Can you work these out from the model? Positions are in its coordinate system, mm. Give positions to 0.01 mm unless a question says otherwise; leave off trailing zeros. Write each loop counter-clockwise with the first axis right and the second up, starting at its lowest first coordinate (ties: lowest second). Pieces come first, ordered by that corner, then holes. Notation, with made-up numbers: (-6, 84) - (-2, 84) arc R28 cw to (-2, 121) - close; hole circle Ø9 at (59.25, 24). An arc over 180 degrees is marked (long way). Return JSON: item names as keys, results as strings. Group by question number.
from build123d import *

# Parameters (mm, degrees)
ESBO_O1_W                = 120
ESBO_O1_H                = 190
RESSALTO_EXTRUS_O1_DEPTH = 2
ESBO_O2_R                = 1
CORTE_EXTRUS_O1_DEPTH    = 10
ESBO_O3_R                = 1
CORTE_EXTRUS_O2_DEPTH    = 113.378823628
FILETE1_R                = 5
ESBO_O4_W                = 3
ESBO_O4_H                = 150
CORTE_EXTRUS_O3_DEPTH    = 113.378823628
FILETE2_R                = 1.5
CORTE_EXTRUS_O4_DEPTH    = 10
ESBO_O6_R                = 1
CORTE_EXTRUS_O5_DEPTH    = 10


with BuildPart() as part:
    # Esboço1 → Ressalto-extrusão1 (new body)
    with BuildSketch(Plane(origin=(0, 0, 0), x_dir=(1, 0, 0), z_dir=(0, 1, 0))):
        Rectangle(ESBO_O1_W, ESBO_O1_H)
    extrude(amount=RESSALTO_EXTRUS_O1_DEPTH)

    # Esboço2 → Corte-extrusão1 (cut)
    with BuildSketch(Plane(origin=(0, 2, 0), x_dir=(1, 0, 0), z_dir=(0, 1, 0))):
        with Locations(Location((0, -37.5, 0), (0, 0, 270))):
            Circle(ESBO_O2_R)
        with Locations(Location((0, -52.5, 0), (0, 0, 90))):
            Circle(ESBO_O2_R)
        with Locations(Location((0, 52.5, 0), (0, 0, 270))):
            Circle(ESBO_O2_R)
        with Locations(Location((0, 37.5, 0), (0, 0, 90))):
            Circle(ESBO_O2_R)
    extrude(amount=-CORTE_EXTRUS_O1_DEPTH, mode=Mode.SUBTRACT)

    # Esboço3 → Corte-extrusão2 (cut, through all)
    with BuildSketch(Plane(origin=(0, 2, 0), x_dir=(1, 0, 0), z_dir=(0, 1, 0))):
        with Locations(Location((-55, 90, 0), (0, 0, 270))):
            Circle(ESBO_O3_R)
        with Locations(Location((55, 90, 0), (0, 0, 90))):
            Circle(ESBO_O3_R)
        with Locations(Location((55, -90, 0), (0, 0, 270))):
            Circle(ESBO_O3_R)
        with Locations(Location((-55, -90, 0), (0, 0, 90))):
            Circle(ESBO_O3_R)
    extrude(amount=-CORTE_EXTRUS_O2_DEPTH, mode=Mode.SUBTRACT)

    # Filete1
    filete1_edges = [part.edges().sort_by_distance(p)[0] for p in [
        (60, 1, 95),
        (-60, 1, 95),
        (-60, 1, -95),
        (60, 1, -95),
    ]]
    fillet(filete1_edges, radius=FILETE1_R)

    # Esboço4 → Corte-extrusão3 (cut, through all)
    with BuildSketch(Plane(origin=(0, 2, 0), x_dir=(1, 0, 0), z_dir=(0, 1, 0))):
        with Locations((58.5, 0)):
            Rectangle(ESBO_O4_W, ESBO_O4_H)
    corte_extrus_o3 = extrude(amount=-CORTE_EXTRUS_O3_DEPTH, mode=Mode.SUBTRACT)

    # Espelhar1: Corte-extrusão3 across plane
    add(corte_extrus_o3.mirror(Plane(origin=(0, 0, 0), x_dir=(0, 0, 1), z_dir=(1, 0, 0))), mode=Mode.SUBTRACT)

    # Filete2
    filete2_edges = [part.edges().sort_by_distance(p)[0] for p in [
        (57, 1, 75),
        (57, 1, -75),
        (-57, 1, 75),
        (-57, 1, -75),
    ]]
    fillet(filete2_edges, radius=FILETE2_R)
    filete2_2_edges = [part.edges().sort_by_distance(p)[0] for p in [
        (60, 1, 75),
        (60, 1, -75),
        (-60, 1, 75),
        (-60, 1, -75),
    ]]
    fillet(filete2_2_edges, radius=FILETE2_R - 0.0001)  # a hair under: the kernel refuses the full size

    # Esboço5 → Corte-extrusão4 (cut)
    with BuildSketch(Plane.XZ):
        with BuildLine():
            Line((-8, 25.5), (8, 25.5))
            ThreePointArc((8, 25.5), (9.414213562, 24.914213562), (10, 23.5))
            Line((10, 23.5), (10, 22.5))
            ThreePointArc((10, 22.5), (9.414213562, 21.085786438), (8, 20.5))
            Line((8, 20.5), (-8, 20.5))
            ThreePointArc((-8, 20.5), (-9.414213562, 21.085786438), (-10, 22.5))
            Line((-10, 22.5), (-10, 23.5))
            ThreePointArc((-10, 23.5), (-9.414213562, 24.914213562), (-8, 25.5))
        make_face()
        with BuildLine():
            Line((10, -23.5), (10, -22.5))
            ThreePointArc((10, -22.5), (9.414213562, -21.085786438), (8, -20.5))
            Line((8, -20.5), (-8, -20.5))
            ThreePointArc((-8, -20.5), (-9.414213562, -21.085786438), (-10, -22.5))
            Line((-10, -22.5), (-10, -23.5))
            ThreePointArc((-10, -23.5), (-9.414213562, -24.914213562), (-8, -25.5))
            Line((-8, -25.5), (8, -25.5))
            ThreePointArc((8, -25.5), (9.414213562, -24.914213562), (10, -23.5))
        make_face()
    extrude(amount=-CORTE_EXTRUS_O4_DEPTH, mode=Mode.SUBTRACT)

    # Esboço6 → Corte-extrusão5 (cut)
    with BuildSketch(Plane.XZ):
        with Locations(Location((9.5, 87, 0), (0, 0, 270))):
            Circle(ESBO_O6_R)
        with Locations(Location((9.5, 71.5, 0), (0, 0, 270))):
            Circle(ESBO_O6_R)
        with Locations(Location((-9.5, 87, 0), (0, 0, 270))):
            Circle(ESBO_O6_R)
        with Locations(Location((-9.5, 71.5, 0), (0, 0, 270))):
            Circle(ESBO_O6_R)
        with BuildLine():
            Line((-5, 86), (5, 86))
            ThreePointArc((5, 86), (6.414213562, 85.414213562), (7, 84))
            Line((7, 84), (7, 80))
            ThreePointArc((7, 80), (6.414213562, 78.585786438), (5, 78))
            Line((5, 78), (-5, 78))
            ThreePointArc((-5, 78), (-6.414213562, 78.585786438), (-7, 80))
            Line((-7, 80), (-7, 84))
            ThreePointArc((-7, 84), (-6.414213562, 85.414213562), (-5, 86))
        make_face()
    corte_extrus_o5 = extrude(amount=-CORTE_EXTRUS_O5_DEPTH, mode=Mode.SUBTRACT)

    # Espelhar2: Corte-extrusão5 across plane
    add(corte_extrus_o5.mirror(Plane.XY), mode=Mode.SUBTRACT)


solid = part.part
1) Will this pin go through, and if not, where does the flat tip stop? pin 1 Ø1 at (y, z) = (1.5, 67) entering from +X.
2) Imagine slicing it at B-B, the plane z = -66.5. Write out the boundary of the cut face in (x, y), and give its area (3 significant figures).
3) I need wall thicknesses on line 1 along X through (y, z) = (1.4, 71.5); line 2 along X through (y, z) = (1.45, -87); line 3 along Z through (x, y) = (-7.5, 1). Which ranges of each line are inside material? Lowest first, please.
4) Imagine slicing it at A-A, the plane y = 1.2. Count the separate pieces of the cut face and the enclosed holes in it, and give its area (3 significant figures).
Resolved:
{
 "1": {"pin 1": "x = 57"},
 "2": {"outline": "(-57, 0) - (57, 0) - (57, 2) - (-57, 2) - close", "area": "228 mm^2"},
 "3": {"line 1": "-57 to -10.5, -8.5 to 8.5, 10.5 to 57", "line 2": "-60 to -10.5, -8.5 to 8.5, 10.5 to 60", "line 3": "-95 to -25.5, -20.5 to 20.5, 25.5 to 95"},
 "4": {"separate pieces": "1", "enclosed holes": "20", "area": "21,400 mm^2"}
}
